Autodesk Inventor part; units mm, degrees
ref_plane "YZ Plane" through (0, 0, 0) normal (1, 0, 0) x (0, 1, 0)
ref_plane "XZ Plane" through (0, 0, 0) normal (0, 1, 0) x (-1, 0, 0)
ref_plane "XY Plane" through (0, 0, 0) normal (0, 0, 1) x (1, 0, 0)
sketch "Sketch1" plane through (0, 0, 0) normal (0, 0, 1) x (1, 0, 0)
  line L0 (-41.9595, 102.9157) -> (590.5005, 102.9157)
  line L1 (590.5005, 102.9157) -> (590.5005, 712.5157)
  line L2 (590.5005, 712.5157) -> (-41.9595, 712.5157)
  line L3 (-41.9595, 712.5157) -> (-41.9595, 102.9157)
  line L4 (-41.9595, 712.5157) -> (-23.3159, 712.5157)
  line L5 (590.5005, 712.5157) -> (546.0505, 712.5157)
  line L6 (546.0505, 712.5157) -> (406.3505, 712.5157)
  line L7 (406.3505, 712.5157) -> (393.6505, 712.5157)
  line L8 (393.6505, 712.5157) -> (253.9505, 712.5157)
  line L9 (253.9505, 712.5157) -> (241.2505, 712.5157)
  line L10 (241.2505, 712.5157) -> (101.5505, 712.5157)
  line L11 (101.5505, 712.5157) -> (88.8505, 712.5157)
  line L12 (88.8505, 712.5157) -> (-23.3159, 712.5157)
  line L13 (590.5005, 102.9157) -> (590.5005, 229.9157)
  line L14 (590.5005, 229.9157) -> (590.5005, 369.6157)
  line L15 (590.5005, 369.6157) -> (590.5005, 382.3157)
  line L16 (590.5005, 382.3157) -> (590.5005, 522.0157)
  circle A0 centre (46.5341, 452.1657) radius 17.4625
  circle A1 centre (198.9341, 452.1657) radius 17.4625
  circle A2 centre (351.3341, 452.1657) radius 17.4625
  circle A3 centre (503.7341, 452.1657) radius 17.4625
  circle A4 centre (46.5341, 299.7657) radius 17.4625
  circle A5 centre (198.9341, 299.7657) radius 17.4625
  circle A6 centre (351.3341, 299.7657) radius 17.4625
  circle A7 centre (503.7341, 299.7657) radius 17.4625
  line L17 (-23.3159, 712.5157) -> (116.3841, 712.5157)
  line L18 (116.3841, 712.5157) -> (129.0841, 712.5157)
  line L19 (129.0841, 712.5157) -> (268.7841, 712.5157)
  line L20 (268.7841, 712.5157) -> (281.4841, 712.5157)
  line L21 (281.4841, 712.5157) -> (421.1841, 712.5157)
  line L22 (421.1841, 712.5157) -> (433.8841, 712.5157)
  line L23 (433.8841, 712.5157) -> (573.5841, 712.5157)
  dimension "d0" = 632.46
  dimension "d1" = 609.6
  dimension "d2" = 18.6436
  dimension "d24" = 127
  dimension "d25" = 139.7
  dimension "d26" = 12.7
  dimension "d27" = 139.7
  dimension "d28" = 34.925
  dimension "d29" = 34.925
  dimension "d30" = 34.925
  dimension "d31" = 34.925
  dimension "d32" = 34.925
  dimension "d33" = 34.925
  dimension "d34" = 34.925
  dimension "d35" = 34.925
  dimension "d38" = 139.7
  dimension "d39" = 12.7
  dimension "d40" = 139.7
  dimension "d41" = 12.7
  dimension "d42" = 139.7
  dimension "d43" = 12.7
  dimension "d44" = 139.7
extrude "Extrusion2" add sketch "Sketch1" along normal blind 6.35
equation "\"BendRadius\" = Thickness"
equation "\"BendReliefWidth\" = Thickness"
equation "\"BendReliefDepth\" = 0.5 * Thickness"
equation "\"CornerReliefSize\" = 4 * Thickness"
equation "\"MinimumRemnant\" = 2 * Thickness"
equation "\"TransitionRadius\" = BendRadius"
equation "\"JacobiRadiusSize\" = BendRadius"
equation "\"GapSize\" = Thickness"
properties part number "vessel support bottom"
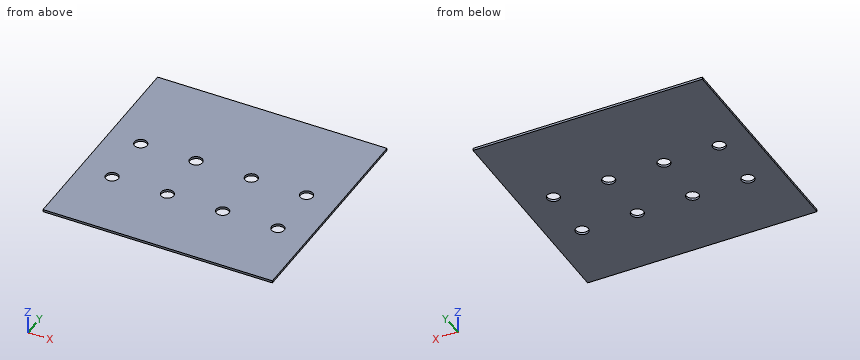
Part model, mm, in its own coordinate system. Round coordinates to 2 decimals unless told otherwise and drop trailing zeros. Loops run counter-clockwise (first coordinate to the right, second up) from the corner with the lowest first, then second, coordinate; pieces in that order, holes last.
Item 1: Drill centre lines: line 1 (Y direction, x = 511, z = 1); line 2 (Y direction, x = 208.5, z = 5.75). Where is each one in solid material? Low to high.
Item 2: Cut at A-A, the plane x = 41. Give the cut face in (y, z).
Item 3: Cut at B-B, the plane z = 3.5. State how many separate pieces and enclosed holes the cut face has, then the cut area to 3 significant figures.
Item 4: Drop a flat-ended pin along its axis: P1, Ø10, axis at x = 94, y = 555.5, coming from the -Z side. Give the stop position or say it passes through.
A:
1. line 1: y = 102.92 to 283.89, 315.64 to 436.29, 468.04 to 712.52
1. line 2: y = 102.92 to 285.16, 314.38 to 437.56, 466.78 to 712.52
2. outline: (102.92, 0) - (283.2, 0) - (283.2, 6.35) - (102.92, 6.35) - close; (316.33, 0) - (435.6, 0) - (435.6, 6.35) - (316.33, 6.35) - close; (468.73, 0) - (712.52, 0) - (712.52, 6.35) - (468.73, 6.35) - close
3. separate pieces: 1
3. enclosed holes: 8
3. area: 378,000 mm2
4. P1: stops at z = 0
